Work out the finished part from the listing and answer in its coordinate system (mm). A direction names the side the tool comes from. Give positions to 0.01 mm unless a question says otherwise; leave off trailing zeros. Loops run counter-clockwise (first coordinate to the right, second up) from the corner with the lowest first, then second, coordinate; pieces in that order, holes last. Notation, with made-up numbers: M -32.75,-31 L -15.75,-31 A18 ccw -15.75,-9 Z; hole C 47.25,5.25 d6. An arc over 180 degrees is marked long. Answer in a Markdown table with one row per item. Add a question column.
from build123d import *

# Parameters (mm, degrees)
EXTRUDE_1_DEPTH          = 4
SKETCH_2_W               = 1.5
SKETCH_2_H               = 6
CUT_EXTRUDE_1_DEPTH      = 15
SKETCH_3_W               = 1
SKETCH_3_H               = 2
CUT_EXTRUDE_2_DEPTH      = 1
CUT_EXTRUDE_2_DEPTH_BACK = 21


with BuildPart() as part:
    # 草图1 → 凸台-拉伸1 (new body)
    with BuildSketch(Plane.XY):
        with BuildLine():
            Line((-14, 20), (0, 20))
            Line((0, 20), (0, 0))
            Line((0, 0), (-1.803847577, 0))
            ThreePointArc((-1.803847577, 0), (-7, 3), (-12.196152423, 0))
            Line((-12.196152423, 0), (-14, 0))
            Line((-14, 0), (-14, 20))
        make_face()
    extrude(amount=EXTRUDE_1_DEPTH)

    # 草图2 → 切除-拉伸1 (cut, through all)
    with BuildSketch(Plane(origin=(0, 0, 0), x_dir=(0, 0, -1), z_dir=(1, 0, 0))):
        with Locations((-0.75, 3)):
            Rectangle(SKETCH_2_W, SKETCH_2_H)
    extrude(amount=-CUT_EXTRUDE_1_DEPTH, mode=Mode.SUBTRACT)

    # 草图3 → 切除-拉伸2 (cut, two sides)
    with BuildSketch(Plane(origin=(0, 20, 0), x_dir=(1, 0, 0), z_dir=(0, 1, 0))) as cut_extrude_2_sk:
        with Locations((-0.5, -2)):
            Rectangle(SKETCH_3_W, SKETCH_3_H)
        with Locations((-13.5, -2)):
            Rectangle(SKETCH_3_W, SKETCH_3_H)
    extrude(amount=CUT_EXTRUDE_2_DEPTH, mode=Mode.SUBTRACT)
    extrude(cut_extrude_2_sk.sketch, amount=-CUT_EXTRUDE_2_DEPTH_BACK, mode=Mode.SUBTRACT)


solid = part.part
(1) Section D-D, the plane y = 12.75 is taken. Determine the outline of the cut face in (x, z).
(2) Section C-C, the plane x = -1.25 is taken. Determine the outline of the cut face in (y, z), and give its area (3 significant figures).
(3) Section A-A, the plane y = 3.5 is taken. Determine the outline of the cut face in (x, z).
(4) Consider line 1 along Z through (x, y) = (-4.75, 3.25); line 2 along Y through (x, z) = (-12.75, 0.8); line 3 along X through (y, z) = (10.25, 1.95). Determine where each line is inside the solid, lowest interval first. Write a range as from..to.
(5) Each of these flat-tipped pins is pushed along its axis until it touches: P1, Ø1.5, axis at x = -3.5, z = 0.5, coming from the -Y side; P2, Ø0.6, axis at y = 9, z = 2, coming from the -X side; P3, Ø3, axis at x = -2, y = 2.5, coming from the -Z side; P4, Ø0.8, axis at x = -13.5, y = 10, coming from the -Z side. Where does it stop, or does it pass through?
(6) Section B-B, the plane z = 2.7 is taken. Determine the outline of the cut face in (x, y).
(7) The mould has two halves that part along Z. Classify faces 6 (the face through (-13.5, 10.1, 3)), 7 (the face through (-1, 10, 2)), 8 (the face through (-7, 4, 1.5)), 9 (the face through (-7, 10, 4)): pulls with the +Z half, pulls with the -Z half, needs draft (parallel to the pull), parting line crosses it, or undercut.
(8) Which of the six approach directions +Z, -Z, +X, -X, +Y, -Y give full straight-line access (tool end or side, diameter ignored) to faces 1 (the face through (-7, 13, 0)), 2 (the face through (-7, 6, 1)), 3 (the face through (0, 13.1, 0.5)), 4 (the face through (-0.5, 10.1, 3)), 5 (the face through (-13.5, 13.1, 1))?
Numbers:
| question | item | result |
|---|---|---|
| 1 | outline | M -14,0 L 0,0 L 0,1 L -1,1 L -1,3 L 0,3 L 0,4 L -14,4 L -14,3 L -13,3 L -13,1 L -14,1 Z |
| 2 | outline | M 0,1.5 L 6,1.5 L 6,0 L 20,0 L 20,4 L 0,4 Z |
| 2 | area | 71.0 mm² |
| 3 | outline | M -14,3 L -13,3 L -13,1.5 L -1,1.5 L -1,3 L 0,3 L 0,4 L -14,4 Z |
| 4 | line 1 | z = 1.5..4 |
| 4 | line 2 | y = 6..20 |
| 4 | line 3 | x = -13..-1 |
| 5 | P1 | stops at y = 6 |
| 5 | P2 | stops at x = -13 |
| 5 | P3 | stops at z = 1.5 |
| 5 | P4 | stops at z = 0 |
| 6 | outline | M -13,0 L -12.2,0 A6 cw -1.8,0 L -1,0 L -1,20 L -13,20 Z |
| 7 | face 6 | undercut |
| 7 | face 7 | undercut |
| 7 | face 8 | pulls with the -Z half |
| 7 | face 9 | pulls with the +Z half |
| 8 | face 1 | -Z, +X, -X, +Y, -Y |
| 8 | face 2 | -Z, +X, -X, -Y |
| 8 | face 3 | +Z, -Z, +X, +Y, -Y |
| 8 | face 4 | +X, +Y, -Y |
| 8 | face 5 | -X, +Y, -Y |
